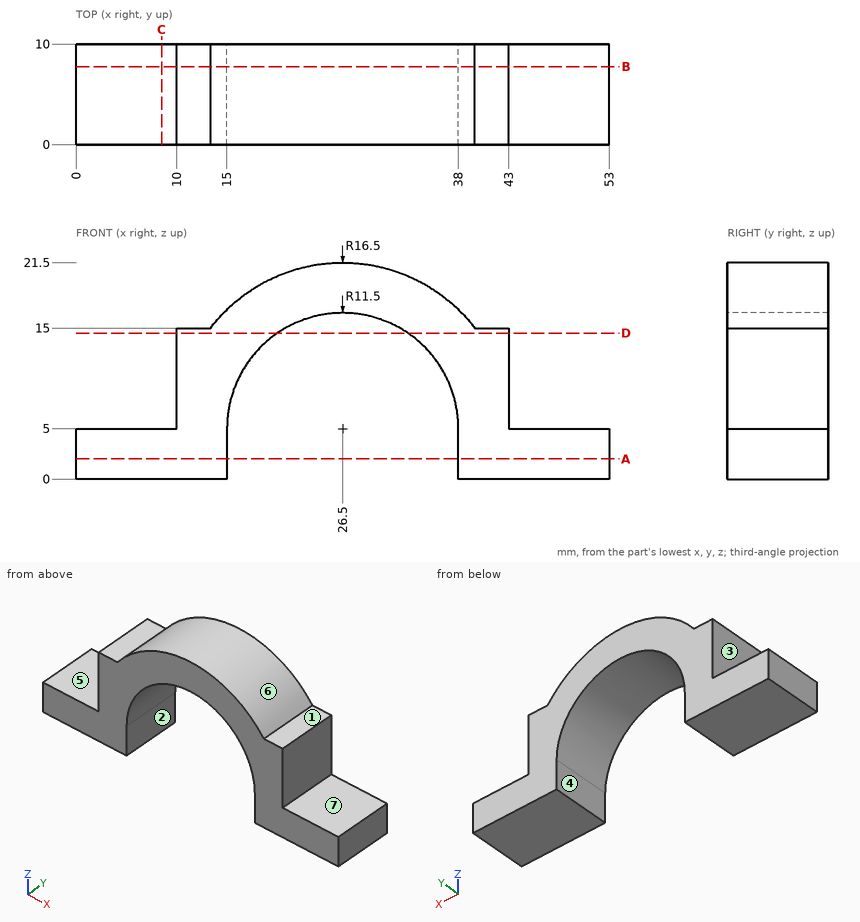
Geometry check sheet. Reference: drawing and pictorial views, mm from the part's lowest x, y, z. A direction names the side the tool comes from. Give positions to 0.01 mm unless a question says otherwise; leave off trailing zeros. Write each loop counter-clockwise with the first axis right and the second up, starting at its lowest first coordinate (ties: lowest second). Pieces come first, ordered by that corner, then holes. Notation, with made-up numbers: (-15, -33.5) -> (23, -33.5) arc R16 cw to (23, -7.5) -> close; hole circle Ø8 at (61.25, 12). An arc over 180 degrees is marked (long way). One line per item, written item: value. Start each with the question number.
Item 1: Tool access check on the marked faces 5, 6 and 7. Record the directions out of +Z, -Z, +X, -X, +Y, -Y that give a thin tool (end or side, any length) a straight path to the whole face; none if there is none.
Item 2: Section check B-B on y = 7.75. Record the cut outline in (x, z).
Item 3: Section check C-C on x = 8.5. Record the cut outline in (y, z), then the cut area to 3 significant figures.
Item 4: Section check A-A on z = 2. Record the cut outline in (x, y).
Item 5: Draft check along X on the marked faces 1, 2, 3 and 4. Enter one of: +X half, -X half, draft (parallel to the pull), parting line (faces both ways), or undercut.
Item 6: Material ranges on probe 1 along X at (y, z) = (2.25, 2); probe 2 along Z at (x, y) = (43.5, 1.75); probe 3 along X at (y, z) = (0.5, 10), recorded low to high. Write a range as from..to.
Item 7: Section check D-D on z = 14.5. Record the cut outline in (x, y).
Item 8: Gauge pin test, flat ends, axial feed: pin 1 (1.7 mm diameter, centred on x = 11.5, y = 3.5, fed in from +Z); pin 2 (3 mm diameter, centred on x = 50.5, y = 3.5, fed in from +Z); pin 3 (5 mm diameter, centred on x = 27.5, y = 4, fed in from -Z). Record the tip position at first contact, or that the pin passes through.
Results list:
1. face 5: +Z, -X, +Y, -Y
1. face 6: +Z, +Y, -Y
1. face 7: +Z, +X, +Y, -Y
2. outline: (0, 0) -> (15, 0) -> (15, 5) arc R11.5 cw to (38, 5) -> (38, 0) -> (53, 0) -> (53, 5) -> (43, 5) -> (43, 15) -> (39.62, 15) arc R16.5 ccw to (13.38, 15) -> (10, 15) -> (10, 5) -> (0, 5) -> close
3. outline: (0, 0) -> (10, 0) -> (10, 5) -> (0, 5) -> close
3. area: 50.0 mm²
4. outline: (0, 0) -> (15, 0) -> (15, 10) -> (0, 10) -> close; (38, 0) -> (53, 0) -> (53, 10) -> (38, 10) -> close
5. face 1: draft
5. face 2: undercut
5. face 3: -X half
5. face 4: undercut
6. probe 1: 0..15, 38..53
6. probe 2: 0..5
6. probe 3: 10..16.14, 36.86..43
7. outline: (10, 0) -> (20.02, 0) -> (20.02, 10) -> (10, 10) -> close; (32.98, 0) -> (43, 0) -> (43, 10) -> (32.98, 10) -> close
8. pin 1: z = 15
8. pin 2: z = 5
8. pin 3: z = 15.95
